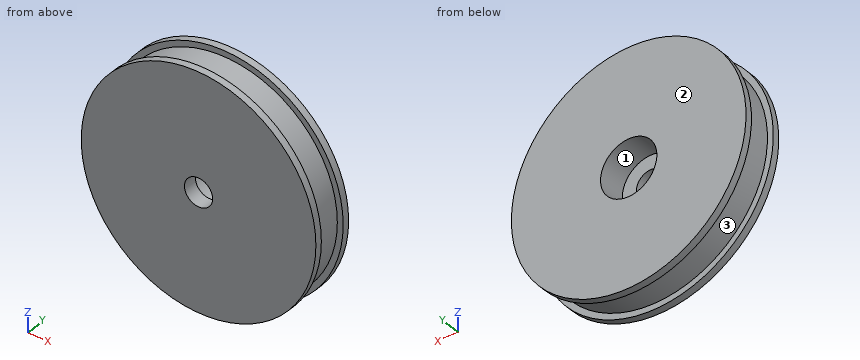
```python
from build123d import *

# Parameters (mm, degrees)
SKETCH1_R           = 12.7
BOSS_EXTRUDE1_DEPTH = 0.762
SKETCH2_R           = 12.065
BOSS_EXTRUDE2_DEPTH = 3.048
SKETCH3_R           = 12.7
BOSS_EXTRUDE3_DEPTH = 0.762
SKETCH4_R           = 3.048
CUT_EXTRUDE1_DEPTH  = 3.048
SKETCH5_R           = 1.524
CUT_EXTRUDE2_DEPTH  = 2.524


with BuildPart() as part:
    # Sketch1 → Boss-Extrude1 (new body)
    with BuildSketch(Plane(origin=(0, 0, 0), x_dir=(1, 0, 0), z_dir=(0, 1, 0))):
        Circle(SKETCH1_R)
    extrude(amount=BOSS_EXTRUDE1_DEPTH)

    # Sketch2 → Boss-Extrude2 (add)
    with BuildSketch(Plane(origin=(0, 0.762, 0), x_dir=(1, 0, 0), z_dir=(0, 1, 0))):
        Circle(SKETCH2_R)
    extrude(amount=BOSS_EXTRUDE2_DEPTH)

    # Sketch3 → Boss-Extrude3 (add)
    with BuildSketch(Plane(origin=(0, 3.81, 0), x_dir=(1, 0, 0), z_dir=(0, 1, 0))):
        Circle(SKETCH3_R)
    extrude(amount=BOSS_EXTRUDE3_DEPTH)

    # Sketch4 → Cut-Extrude1 (cut)
    with BuildSketch(Plane(origin=(0, 4.572, 0), x_dir=(1, 0, 0), z_dir=(0, 1, 0))):
        Circle(SKETCH4_R)
    extrude(amount=-CUT_EXTRUDE1_DEPTH, mode=Mode.SUBTRACT)

    # Sketch5 → Cut-Extrude2 (cut, through all)
    with BuildSketch(Plane(origin=(0, 1.524, 0), x_dir=(1, 0, 0), z_dir=(0, 1, 0))):
        Circle(SKETCH5_R)
    extrude(amount=-CUT_EXTRUDE2_DEPTH, mode=Mode.SUBTRACT)


solid = part.part
```
Can you work these out from the model? Positions are in its coordinate system, mm. Face numbers are marked on the shaded views. Coordinates: 2 decimals unless noted, no trailing zeros. Loops run counter-clockwise (first coordinate to the right, second up) from the corner with the lowest first, then second, coordinate; pieces in that order, holes last. Notation, with made-up numbers: M 65,86.25 L 71,86.25 A20 cw 71,109.25 Z; hole C 3,-37.75 d3. An arc over 180 degrees is marked long. Put each result on its own line as item: value. Start each with the question number.
(1) Imagine slicing it at D-D on z = 10. List the corners of the cut face in (x, y) for me, and give its area (3 significant figures).
(2) I need wall thicknesses on probe 1 along X at (y, z) = (1, 0) (3 decimals); probe 2 along X at (y, z) = (3.25, 0) (3 decimals). Which ranges of each line are inside material? Lowest first, please.
(3) Imagine slicing it at C-C on y = 0.45. List the corners of the cut face in (x, z) for me.
(4) Imagine slicing it at B-B on x = 0. List the corners of the cut face in (y, z) for me (3 decimals).
(5) Will these pins go through, and if not, where does the flat tip stop? pin 1 Ø1 at (x, y) = (-0.5, 2.5) entering from -Z (3 decimals); pin 2 Ø2 at (x, y) = (0.5, 2.5) entering from +Z (3 decimals); pin 3 Ø5 at (x, z) = (0.5, 0) entering from +Y; pin 4 Ø2.5 at (x, z) = (0, 0) entering from -Y.
(6) Imagine slicing it at A-A on z = 0. List the corners of the cut face in (x, y) for me (3 decimals).
(7) We'd pull the mould along X, two halves only. Please class the marked faces 1, 2 and 3: +X half, -X half, draft (parallel to the pull), parting line (faces both ways), or undercut.
Worked answers:
1. outline: M -7.83,0 L 7.83,0 L 7.83,0.76 L 6.75,0.76 L 6.75,3.81 L 7.83,3.81 L 7.83,4.57 L -7.83,4.57 L -7.83,3.81 L -6.75,3.81 L -6.75,0.76 L -7.83,0.76 Z
1. area: 65.0 mm2
2. probe 1: x = -12.065 to -1.524, 1.524 to 12.065
2. probe 2: x = -12.065 to -3.048, 3.048 to 12.065
3. outline: C 0,0 d25.4; hole C 0,0 d3.05
4. outline: M 0,-12.7 L 0.762,-12.7 L 0.762,-12.065 L 3.81,-12.065 L 3.81,-12.7 L 4.572,-12.7 L 4.572,-3.048 L 1.524,-3.048 L 1.524,-1.524 L 0,-1.524 Z; M 0,1.524 L 1.524,1.524 L 1.524,3.048 L 4.572,3.048 L 4.572,12.7 L 3.81,12.7 L 3.81,12.065 L 0.762,12.065 L 0.762,12.7 L 0,12.7 Z
5. pin 1: stops at z = -12.065
5. pin 2: stops at z = 12.065
5. pin 3: stops at y = 1.52
5. pin 4: passes through
6. outline: M -12.7,0 L -1.524,0 L -1.524,1.524 L -3.048,1.524 L -3.048,4.572 L -12.7,4.572 L -12.7,3.81 L -12.065,3.81 L -12.065,0.762 L -12.7,0.762 Z; M 1.524,0 L 12.7,0 L 12.7,0.762 L 12.065,0.762 L 12.065,3.81 L 12.7,3.81 L 12.7,4.572 L 3.048,4.572 L 3.048,1.524 L 1.524,1.524 Z
7. face 1: undercut
7. face 2: draft
7. face 3: parting line
